```python
from build123d import *

# Parameters (mm, degrees)
SKETCH1_W                  = 431.8
SKETCH1_H                  = 171.45
BOSS_EXTRUDE1_DEPTH        = 85.725
CUT_EXTRUDE1_DEPTH         = 73.025
FILLET3_R                  = 44.45
F_0_25_OFF_THE_TOP_DEPTH   = 6.35
SKETCH4_W                  = 431.8
SKETCH4_H                  = 79.375
F_0_12_OFF_THE_SIDE_DEPTH  = 2.54
SKETCH5_W                  = 168.91
SKETCH5_H                  = 79.375
F_0_12_OFF_THE_FRONT_DEPTH = 3.048
SKETCH6_W                  = 428.752
SKETCH6_H                  = 79.375
CUT_EXTRUDE5_DEPTH         = 3.048
SKETCH7_W                  = 165.862
SKETCH7_H                  = 79.375
CUT_EXTRUDE6_DEPTH         = 3.048
FILLET5_R                  = 6.35


with BuildPart() as part:
    # Sketch1 → Boss-Extrude1 (new body)
    with BuildSketch(Plane(origin=(0, 0, 0), x_dir=(1, 0, 0), z_dir=(0, 1, 0))):
        Rectangle(SKETCH1_W, SKETCH1_H)
    extrude(amount=BOSS_EXTRUDE1_DEPTH)

    # Sketch2 → Cut-Extrude1 (cut)
    with BuildSketch(Plane.XZ):
        with BuildLine():
            Line((162.16885638, 76.686434381), (-162.16885638, 76.686434381))
            ThreePointArc((-162.16885638, 76.686434381), (-193.771281353, 63.596281353), (-206.861434381, 31.99385638))
            Line((-206.861434381, 31.99385638), (-206.861434381, -31.99385638))
            ThreePointArc((-206.861434381, -31.99385638), (-193.771281353, -63.596281353), (-162.16885638, -76.686434381))
            Line((-162.16885638, -76.686434381), (162.16885638, -76.686434381))
            ThreePointArc((162.16885638, -76.686434381), (193.771281353, -63.596281353), (206.861434381, -31.99385638))
            Line((206.861434381, -31.99385638), (206.861434381, 31.99385638))
            ThreePointArc((206.861434381, 31.99385638), (193.771281353, 63.596281353), (162.16885638, 76.686434381))
        make_face()
    extrude(amount=-CUT_EXTRUDE1_DEPTH, mode=Mode.SUBTRACT)

    # Fillet3
    fillet3_edges = [part.edges().sort_by_distance(p)[0] for p in [
        (215.9, 42.8625, 85.725),
        (-215.9, 42.8625, 85.725),
        (-215.9, 42.8625, -85.725),
        (215.9, 42.8625, -85.725),
    ]]
    fillet(fillet3_edges, radius=FILLET3_R)

    # Sketch3 → 0.25 off the top (cut)
    with BuildSketch(Plane(origin=(0, 85.725, 0), x_dir=(1, 0, 0), z_dir=(0, 1, 0))):
        with BuildLine():
            Line((215.9, -41.275), (215.9, 41.275))
            ThreePointArc((215.9, 41.275), (202.880896424, 72.705896424), (171.45, 85.725))
            Line((171.45, 85.725), (-171.45, 85.725))
            ThreePointArc((-171.45, 85.725), (-202.880896424, 72.705896424), (-215.9, 41.275))
            Line((-215.9, 41.275), (-215.9, -41.275))
            ThreePointArc((-215.9, -41.275), (-202.880896424, -72.705896424), (-171.45, -85.725))
            Line((-171.45, -85.725), (171.45, -85.725))
            ThreePointArc((171.45, -85.725), (202.880896424, -72.705896424), (215.9, -41.275))
        make_face()
    extrude(amount=-F_0_25_OFF_THE_TOP_DEPTH, mode=Mode.SUBTRACT)

    # Sketch4 → 0.12 off the side (cut)
    with BuildSketch(Plane.XY.offset(85.725)):
        with Locations((0, 39.6875)):
            Rectangle(SKETCH4_W, SKETCH4_H)
    extrude(amount=-F_0_12_OFF_THE_SIDE_DEPTH, mode=Mode.SUBTRACT)

    # Sketch5 → 0.12 off the front (cut)
    with BuildSketch(Plane.ZY.offset(215.9)):
        with Locations((-1.27, 39.6875)):
            Rectangle(SKETCH5_W, SKETCH5_H)
    extrude(amount=-F_0_12_OFF_THE_FRONT_DEPTH, mode=Mode.SUBTRACT)

    # Sketch6 → Cut-Extrude5 (cut)
    with BuildSketch(Plane(origin=(0, 0, -85.725), x_dir=(-1, 0, 0), z_dir=(0, 0, -1))):
        with Locations((-1.524, 39.6875)):
            Rectangle(SKETCH6_W, SKETCH6_H)
    extrude(amount=-CUT_EXTRUDE5_DEPTH, mode=Mode.SUBTRACT)

    # Sketch7 → Cut-Extrude6 (cut)
    with BuildSketch(Plane(origin=(215.9, 0, 0), x_dir=(0, 0, -1), z_dir=(1, 0, 0))):
        with Locations((-0.254, 39.6875)):
            Rectangle(SKETCH7_W, SKETCH7_H)
    extrude(amount=-CUT_EXTRUDE6_DEPTH, mode=Mode.SUBTRACT)

    # Fillet5
    fillet5_edges = [part.edges().sort_by_distance(p)[0] for p in [
        (-212.852, 79.375, 0),
        (0, 79.375, -82.677),
        (212.852, 79.375, 0),
        (0, 79.375, 83.185),
    ]]
    fillet(fillet5_edges, radius=FILLET5_R)


solid = part.part
```
CAD build for the part. Positions are in the model's coordinates, mm. A direction names the side the tool comes from. Round coordinates to 2 decimals unless told otherwise and drop trailing zeros. Order: outer loops, then holes, each group sorted by start corner. A loop starts at its lowest first (then second) coordinate and runs counter-clockwise, first axis right, second up. Notation, with made-up numbers: (-16, 55.5) - (6, 55.5) arc R27 ccw to (6, 89.5) - close; hole circle Ø5 at (71.25, 46.25). An arc over 180 degrees is marked (long way). Answer in a Markdown table with one row per item. Add a question column.
(1) Mould opens along Z. For faces 3 (the face through (-203.062, 40.243, -72.524)), 4 (the face through (212.852, 37, 1)), 5 (the face through (-2, 36, -76.686)) say: +Z half, -Z half, draft (parallel to the pull), parting line (faces both ways), or undercut.
(2) 3-axis set-ups, long thin cutter, end or side, ignore diameter. For faces 1 (the face through (2, 36, 76.686)), 2 (the face through (-212.852, 37, -1)): which of +Z, -Z, +X, -X, +Y, -Y reach the whole face in a straight line?
(3) Probe L1, parallel to Z at x = -37, y = 33.5 (3 decimals); L2, parallel to X at y = 70, z = 30.5; L3, parallel to X at y = 66.5, z = 33. List the from-to ranges inside material, lowest first. Write a range as [from, to].
(4) Band-saw the part on A-A on y = 31. List the corners of the cut face in (x, z) (3 decimals), and give its area (3 significant figures).
(5) Band-saw the part on C-C on x = -97. List the corners of the cut face in (y, z) (3 decimals).
(6) Band-saw the part on B-B on z = 24.5. List the corners of the cut face in (x, y) (3 decimals), and give its area (3 significant figures).
Data:
| question | item | result |
|---|---|---|
| 1 | face 3 | -Z half |
| 1 | face 4 | draft |
| 1 | face 5 | undercut |
| 2 | face 1 | -Y |
| 2 | face 2 | +Z, -Z, -X, +Y, -Y |
| 3 | L1 | z = [-82.677, -76.686], [76.686, 83.185] |
| 3 | L2 | x = [-212.85, -206.86], [206.86, 212.85] |
| 3 | L3 | x = [-212.85, -206.85], [206.85, 212.85] |
| 4 | outline | (-212.852, -57.451) arc R44.45 ccw to (-187.626, -82.677) - (187.626, -82.677) arc R44.45 ccw to (212.852, -57.451) - (212.852, 57.451) arc R44.45 ccw to (186.261, 83.185) - (-186.261, 83.185) arc R44.45 ccw to (-212.852, 57.451) - close; hole (-206.861, -31.994) arc R44.693 ccw to (-162.169, -76.686) - (162.169, -76.686) arc R44.693 ccw to (206.861, -31.994) - (206.861, 31.994) arc R44.693 ccw to (162.169, 76.686) - (-162.169, 76.686) arc R44.693 ccw to (-206.861, 31.994) - close |
| 4 | area | 7,930 mm^2 |
| 5 | outline | (0, -82.677) - (73.025, -82.677) arc R6.35 ccw to (79.375, -76.327) - (79.375, 76.835) arc R6.35 ccw to (73.025, 83.185) - (0, 83.185) - (0, 76.686) - (73.025, 76.686) - (73.025, -76.686) - (0, -76.686) - close |
| 6 | outline | (-212.852, 0) - (-206.861, 0) - (-206.861, 73.025) - (206.861, 73.025) - (206.861, 0) - (212.852, 0) - (212.852, 73.025) arc R6.35 ccw to (206.502, 79.375) - (-206.502, 79.375) arc R6.35 ccw to (-212.852, 73.025) - close |
| 6 | area | 3,560 mm^2 |
